from build123d import *

# Parameters (mm, degrees)
SKETCH3_R                                    = 114.3
SKETCH3_R_2                                  = 73.533
BOSS_EXTRUDE1_DEPTH                          = 12.7
SKETCH16_R                                   = 19.05
BOSS_EXTRUDE2_DEPTH                          = 12.7
CIRPATTERN6_COUNT                            = 4
CIRPATTERN2_COUNT                            = 20
F_1_4_20_TAPPED_HOLE2_D                      = 5.1054
CIRPATTERN4_COUNT                            = 20
CBORE_FOR_1_4_BINDING_HEAD_MACHINE_S_2_COUNT = 2
CBORE_FOR_1_4_BINDING_HEAD_MACHINE_S_2_PITCH = 152.4
CBORE_FOR_1_4_BINDING_HEAD_MACHINE_S_3_COUNT = 2
CBORE_FOR_1_4_BINDING_HEAD_MACHINE_S_3_PITCH = 215.526146906
CBORE_FOR_1_4_BINDING_HEAD_MACHINE_S_4_COUNT = 2
CBORE_FOR_1_4_BINDING_HEAD_MACHINE_S_4_PITCH = 152.4


with BuildPart() as part:
    # Sketch3 → Boss-Extrude1 (new body)
    with BuildSketch(Plane(origin=(0, 0, 0), x_dir=(1, 0, 0), z_dir=(0, 1, 0))):
        Circle(SKETCH3_R)
        Circle(SKETCH3_R_2, mode=Mode.SUBTRACT)
    extrude(amount=BOSS_EXTRUDE1_DEPTH)

    # Sketch16 → Boss-Extrude2 (add)
    with BuildSketch(Plane(origin=(0, 12.7, 0), x_dir=(1, 0, 0), z_dir=(0, 1, 0))):
        with Locations((107.763073453, 0)):
            Circle(SKETCH16_R)
    boss_extrude2 = extrude(amount=-BOSS_EXTRUDE2_DEPTH)

    # CirPattern6: Boss-Extrude2 ×4 about axis
    cirpattern6_axis = Axis((0, 0, 0), (0, 1, 0))
    for i in range(1, CIRPATTERN6_COUNT):
        add(boss_extrude2.rotate(cirpattern6_axis, i * 360 / CIRPATTERN6_COUNT))

    # Sketch8 → CBORE for 5_16 Binding Head Machine Scre (revolve, cut)
    with BuildSketch(Plane(origin=(89.411079645, 12.7, -14.161323808), x_dir=(0, 0, 1), z_dir=(1, 0, 0))):
        Polygon((0, 0), (0, 12.7), (4.2164, 12.7), (4.2164, 5.3086), (8.73125, 5.3086), (8.73125, 0.15875), (8.89, 0), align=None)
    cbore_for_5_16_binding_head_machine_scre = revolve(axis=Axis((89.411079645, 19.05, -14.161323808), (0, -1, 0)), mode=Mode.SUBTRACT)

    # CirPattern2: CBORE for 5_16 Binding Head Machine Scre ×20 about axis
    cirpattern2_axis = Axis((0, 0, 0), (0, 1, 0))
    for i in range(1, CIRPATTERN2_COUNT):
        add(cbore_for_5_16_binding_head_machine_scre.rotate(cirpattern2_axis, i * 360 / CIRPATTERN2_COUNT), mode=Mode.SUBTRACT)

    # 1_4-20 Tapped Hole2 (through all)
    with Locations(Plane(origin=(0, 12.7, 0), x_dir=(1, 0, 0), z_dir=(0, 1, 0))):
        with Locations((78.232, 0)):
            f_1_4_20_tapped_hole2 = Hole(F_1_4_20_TAPPED_HOLE2_D / 2)

    # CirPattern4: 1_4-20 Tapped Hole2 ×20 about axis
    cirpattern4_axis = Axis((0, 0, 0), (0, 1, 0))
    for i in range(1, CIRPATTERN4_COUNT):
        add(f_1_4_20_tapped_hole2.rotate(cirpattern4_axis, i * 360 / CIRPATTERN4_COUNT), mode=Mode.SUBTRACT)

    # Sketch19 → CBORE for 1_4 Binding Head Machine Screw (revolve, cut)
    with BuildSketch(Plane(origin=(0, 0, 107.763073453), x_dir=(0, 0, -1), z_dir=(1, 0, 0))):
        Polygon((0, 0), (0, 12.7), (3.57124, 12.7), (3.57124, 4.191), (7.14375, 4.191), (7.14375, 0.635), (7.77875, 0), align=None)
    cbore_for_1_4_binding_head_machine_screw = revolve(axis=Axis((0, -6.35, 107.763073453), (0, 1, 0)), mode=Mode.SUBTRACT)

    # CBORE for 1_4 Binding Head Machine S 2: CBORE for 1_4 Binding Head Machine Screw ×2
    with Locations(*[Vector(0.707106781, 0, -0.707106781) * (i * CBORE_FOR_1_4_BINDING_HEAD_MACHINE_S_2_PITCH) for i in range(1, CBORE_FOR_1_4_BINDING_HEAD_MACHINE_S_2_COUNT)]):
        add(cbore_for_1_4_binding_head_machine_screw, mode=Mode.SUBTRACT)

    # CBORE for 1_4 Binding Head Machine S 3: CBORE for 1_4 Binding Head Machine Screw ×2
    with Locations(*[(0, 0, -i * CBORE_FOR_1_4_BINDING_HEAD_MACHINE_S_3_PITCH) for i in range(1, CBORE_FOR_1_4_BINDING_HEAD_MACHINE_S_3_COUNT)]):
        add(cbore_for_1_4_binding_head_machine_screw, mode=Mode.SUBTRACT)

    # CBORE for 1_4 Binding Head Machine S 4: CBORE for 1_4 Binding Head Machine Screw ×2
    with Locations(*[Vector(-0.707106781, 0, -0.707106781) * (i * CBORE_FOR_1_4_BINDING_HEAD_MACHINE_S_4_PITCH) for i in range(1, CBORE_FOR_1_4_BINDING_HEAD_MACHINE_S_4_COUNT)]):
        add(cbore_for_1_4_binding_head_machine_screw, mode=Mode.SUBTRACT)


solid = part.part
The listing builds one solid part. Answer for the finished solid, in the listing's coordinates (mm). A direction names the side the tool comes from. Coordinates: 2 decimals unless noted, no trailing zeros. Answer in a Markdown table with one row per item.
1) Find section A-A (z = 14). Count the separate pieces of the cut face and the enclosed holes in it, then the cut area to 3 significant figures.
Answers below:
| item | result |
|---|---|
| separate pieces | 4 |
| enclosed holes | 0 |
| area | 922 mm^2 |
2) Determine the mould class of faces 4 (the cylindrical face through (0.35, 6.44, -126.81)), 5 (the flat face through (40, 7.391, 85)) for opening direction Z: released by +Z, released by -Z, zero draft, split by the parting line, or undercut.
Answers below:
| item | result |
|---|---|
| face 4 | released by -Z |
| face 5 | undercut |
3) Find the intervals of material crossed by probe 1 along Z at (x, y) = (77, 5.5); probe 2 along Z at (x, y) = (12.5, 10.5); probe 3 along Z at (x, y) = (47.5, 8.75), in increasing order.
Answers below:
| item | result |
|---|---|
| probe 1 | -84.47 to -43.19, -39 to -2.24, 2.24 to 39, 43.19 to 84.47 |
| probe 2 | -122.14 to -97.98, -80.84 to -72.46, 72.46 to 80.84, 97.98 to 122.14 |
| probe 3 | -103.96 to -86.6, -74.72 to -65.34, -61.24 to -56.13, 56.13 to 61.24, 65.34 to 74.72, 86.6 to 103.96 |
4) Given pin 1 (13.5 mm diameter, centred on x = -80.66, z = 41.1, fed in from +Y); pin 2 (1 mm diameter, centred on x = 100, y = 5, fed in from +Z); pin 3 (1 mm diameter, centred on x = -58, y = 3, fed in from +Z), each flat-ended and moving along its own axis, determine where each tip first touches the part or whether it passes through.
Answers below:
| item | result |
|---|---|
| pin 1 | y = 7.39 |
| pin 2 | z = 56.25 |
| pin 3 | z = 98.78 |
5) Which of the six approach directions +Z, -Z, +X, -X, +Y, -Y give full straight-line access (tool end or side, diameter ignored) to faces 1 (the cylindrical face through (15.22, 3.75, -85.33)), 2 (the flat face through (37, 7.391, -78)), 3 (the cylindrical face through (-100.79, 2.39, 1.55))?
Answers below:
| item | result |
|---|---|
| face 1 | +Y, -Y |
| face 2 | +Y |
| face 3 | -Y |
